Check sheet for the modelled part. Datum: model origin and axes. Units: mm. Round coordinates to 2 decimals unless told otherwise and drop trailing zeros. Order: outer loops, then holes, each group sorted by start corner. A loop starts at its lowest first (then second) coordinate and runs counter-clockwise, first axis right, second up. Notation, with made-up numbers: (-11, 36) -> (45, 36) arc R29 cw to (45, 70) -> close; hole circle Ø10 at (13, -1). An arc over 180 degrees is marked (long way). Use CSV: the item, a comma, the result in double quotes.
```python
from build123d import *

# Parameters (mm, degrees)
SKETCH1_R                                  = 38.1
SKETCH1_R_2                                = 16
BOSS_EXTRUDE1_DEPTH                        = 25.4
F_10_5_10_5_DIAMETER_HOLE1_D               = 10.5
F_10_5_10_5_DIAMETER_HOLE1_DEPTH           = 300
F_10_5_10_5_DIAMETER_HOLE1_TIP             = 3.15451825
F_10_5_10_5_DIAMETER_HOLE1_ON_FACE_2_D     = 10.5
F_10_5_10_5_DIAMETER_HOLE1_ON_FACE_2_DEPTH = 300
F_10_5_10_5_DIAMETER_HOLE1_ON_FACE_2_TIP   = 3.15451825
F_10_5_10_5_DIAMETER_HOLE1_ON_FACE_3_D     = 10.5
F_10_5_10_5_DIAMETER_HOLE1_ON_FACE_3_DEPTH = 300
F_10_5_10_5_DIAMETER_HOLE1_ON_FACE_3_TIP   = 3.15451825


with BuildPart() as part:
    # Sketch1 → Boss-Extrude1 (new body)
    with BuildSketch(Plane(origin=(0, 0, 0), x_dir=(1, 0, 0), z_dir=(0, 1, 0))):
        Circle(SKETCH1_R)
        Circle(SKETCH1_R_2, mode=Mode.SUBTRACT)
    extrude(amount=BOSS_EXTRUDE1_DEPTH)

    # Ø10.5 (10.5) Diameter Hole1
    with Locations(Plane(origin=(-0.05014739, 13, -38.099966998), x_dir=(-0.999999134, 0, 0.001316204), z_dir=(-0.001316204, 0, -0.999999134))):
        with Locations((0, 0)):
            Hole(F_10_5_10_5_DIAMETER_HOLE1_D / 2, depth=F_10_5_10_5_DIAMETER_HOLE1_DEPTH)
            with Locations((0, 0, -(F_10_5_10_5_DIAMETER_HOLE1_DEPTH + F_10_5_10_5_DIAMETER_HOLE1_TIP / 2))):  # 118° drill point
                Cone(0, F_10_5_10_5_DIAMETER_HOLE1_D / 2, F_10_5_10_5_DIAMETER_HOLE1_TIP, mode=Mode.SUBTRACT)

    # Ø10.5 (10.5) Diameter Hole1 on face 2
    with Locations(Plane(origin=(-38.1, 13, 0), x_dir=(0, 0, -1), z_dir=(-1, 0, 0))):
        with Locations((0, 0)):
            Hole(F_10_5_10_5_DIAMETER_HOLE1_ON_FACE_2_D / 2, depth=F_10_5_10_5_DIAMETER_HOLE1_ON_FACE_2_DEPTH)
            with Locations((0, 0, -(F_10_5_10_5_DIAMETER_HOLE1_ON_FACE_2_DEPTH + F_10_5_10_5_DIAMETER_HOLE1_ON_FACE_2_TIP / 2))):  # 118° drill point
                Cone(0, F_10_5_10_5_DIAMETER_HOLE1_ON_FACE_2_D / 2, F_10_5_10_5_DIAMETER_HOLE1_ON_FACE_2_TIP, mode=Mode.SUBTRACT)

    # Ø10.5 (10.5) Diameter Hole1 on face 3
    with Locations(Plane(origin=(19.117815044, 0, -19.06591587), x_dir=(0, 0, -1), z_dir=(0, -1, 0))):
        with Locations((0, 0), (0, -38.235630088), (-38.13183174, -38.235630088), (-38.13183174, 0)):
            Hole(F_10_5_10_5_DIAMETER_HOLE1_ON_FACE_3_D / 2, depth=F_10_5_10_5_DIAMETER_HOLE1_ON_FACE_3_DEPTH)
            with Locations((0, 0, -(F_10_5_10_5_DIAMETER_HOLE1_ON_FACE_3_DEPTH + F_10_5_10_5_DIAMETER_HOLE1_ON_FACE_3_TIP / 2))):  # 118° drill point
                Cone(0, F_10_5_10_5_DIAMETER_HOLE1_ON_FACE_3_D / 2, F_10_5_10_5_DIAMETER_HOLE1_ON_FACE_3_TIP, mode=Mode.SUBTRACT)


solid = part.part
```
Q1. Sectioned sample at C-C, the plane y = 13. Enter the section's corners in (x, z).
Result sheet:
outline,"(-37.74, -5.25) arc R38.1 ccw to (-5.3, -37.73) -> (-5.27, -15.11) arc R16 cw to (-15.11, -5.25) -> close; (-37.74, 5.25) -> (-15.11, 5.25) arc R16 cw to (-5.23, 15.12) -> (-5.2, 37.74) arc R38.1 ccw to start; (5.2, -37.74) arc R38.1 ccw to (37.74, -5.25) -> (15.11, -5.25) arc R16 cw to (5.23, -15.12) -> close; (5.27, 15.11) arc R16 cw to (15.11, 5.25) -> (37.74, 5.25) arc R38.1 ccw to (5.3, 37.73) -> close; hole circle Ø10.5 at (-19.12, -19.07); hole circle Ø10.5 at (-19.12, 19.07); hole circle Ø10.5 at (19.12, -19.07); hole circle Ø10.5 at (19.12, 19.07)"
Q2. Mould release check, pull along Z, two halves, no side actions. Record for faces 1 (the face through (35.195, 12.522, 14.593)), 2 (the face through (-26.447, 7.795, -0.683)), 3 (the face through (16.4, 0, -0.5)): pulls with the +Z half, pulls with the -Z half, needs draft (parallel to the pull), parting line crosses it, or undercut.
Result sheet:
face 1,"parting line crosses it"
face 2,"undercut"
face 3,"needs draft"
Q3. Scan lines: L1, parallel to Y at x = 28.75, z = 0; L2, parallel to X at y = 24, z = -23.5; L3, parallel to X at y = 22.75, z = 20.5. Record each from-to range of solid material in increasing order.
Result sheet:
L1,"y = 0 to 7.75, 18.25 to 25.4"
L2,"x = -29.99 to -21.93, -16.31 to 16.31, 21.93 to 29.99"
L3,"x = -32.11 to -24.17, -14.07 to 14.07, 24.17 to 32.11"
Q4. Sectioned sample at D-D, the plane x = -30. Enter the section's corners in (y, z), then the cut area to 3 significant figures.
Result sheet:
outline,"(0, -23.49) -> (25.4, -23.49) -> (25.4, 23.49) -> (0, 23.49) -> close; hole circle Ø10.5 at (13, 0)"
area,"1,110 mm^2"
Q5. Sectioned sample at A-A, the plane z = 0. Enter the section's corners in (x, y).
Result sheet:
outline,"(-38.1, 0) -> (-16, 0) -> (-16, 7.75) -> (-38.1, 7.75) -> close; (-38.1, 18.25) -> (-16, 18.25) -> (-16, 25.4) -> (-38.1, 25.4) -> close; (16, 0) -> (38.1, 0) -> (38.1, 7.75) -> (16, 7.75) -> close; (16, 18.25) -> (38.1, 18.25) -> (38.1, 25.4) -> (16, 25.4) -> close"
Q6. Sectioned sample at B-B, the plane x = -20.5. Enter the section's corners in (y, z), then the cut area to 3 significant figures.
Result sheet:
outline,"(0, -32.11) -> (25.4, -32.11) -> (25.4, -24.13) -> (0, -24.13) -> close; (0, -14) -> (25.4, -14) -> (25.4, 14) -> (0, 14) -> close; (0, 24.13) -> (25.4, 24.13) -> (25.4, 32.11) -> (0, 32.11) -> close; hole circle Ø10.5 at (13, 0)"
area,"1,030 mm^2"
Q7. Go/stop test with flat-tipped pins: pin 1 (8.5 mm diameter, centred on x = 19.12, z = -19.07, fed in from +Y); pin 2 (2 mm diameter, centred on y = 8.5, z = 26, fed in from -X); pin 3 (4 mm diameter, centred on y = 5.5, z = 14.5, fed in from -X); pin 4 (1 mm diameter, centred on x = -18, y = 17.5, fed in from +Z). Record where each tip stops, or that it passes through.
Result sheet:
pin 1,"passes through"
pin 2,"stops at x = -28.75"
pin 3,"stops at x = -35.99"
pin 4,"stops at z = 33.84"
